from build123d import *
from OCP.BRepFilletAPI import BRepFilletAPI_MakeChamfer

# Parameters (mm, degrees)
SKETCH1_W                  = 50
SKETCH1_H                  = 180
BOSS_EXTRUDE1_DEPTH        = 6
CHAMFER2_SIZE              = 10
F_3_3_3_3_DIAMETER_HOLE1_D = 3.3
BOSS_EXTRUDE3_DEPTH        = 6
CUT_EXTRUDE3_DEPTH         = 2.2
BOSS_EXTRUDE4_DEPTH        = 6
CHAMFER14_SIZE             = 2
CHAMFER16_SIZE             = 7
CHAMFER16_SIZE_2           = 56.79198309
CHAMFER17_SIZE             = 2
SKETCH59_W                 = 21.7
SKETCH59_H                 = 5
BOSS_EXTRUDE5_DEPTH        = 6
CHAMFER19_SIZE             = 5
CUT_EXTRUDE28_DEPTH        = 106.814167745
CHAMFER20_SIZE             = 3
CHAMFER20_SIZE2            = 3.484649721
CUT_EXTRUDE29_DEPTH        = 105.986313168
CHAMFER24_SIZE             = 1
CUT_EXTRUDE31_DEPTH        = 105.986313306
SKETCH66_R                 = 6
BOSS_EXTRUDE6_DEPTH        = 6


with BuildPart() as part:
    # Sketch1 → Boss-Extrude1 (new body)
    with BuildSketch(Plane(origin=(0, 0, 0), x_dir=(1, 0, 0), z_dir=(0, 1, 0))):
        Rectangle(SKETCH1_W, SKETCH1_H)
    extrude(amount=BOSS_EXTRUDE1_DEPTH)

    # Chamfer2
    chamfer2_edges = [part.edges().sort_by_distance(p)[0] for p in [
        (-25, 3, -90),
        (25, 3, -90),
        (25, 3, 90),
        (-25, 3, 90),
    ]]
    chamfer(chamfer2_edges, length=CHAMFER2_SIZE)

    # Ø3.3 (3.3) Diameter Hole1 (through all)
    with Locations(Plane(origin=(0, 6, 0), x_dir=(1, 0, 0), z_dir=(0, 1, 0))):
        with Locations((-19.785088487, 16.105600012), (9.214911513, -56.894399988), (20.785088487, -43.105600012), (-9.214911513, -56.894399988), (-20.785088487, -43.105600012), (19.785088487, 16.105600012), (8.214911513, 29.894399988), (-8.214911513, 29.894399988)):
            Hole(F_3_3_3_3_DIAMETER_HOLE1_D / 2)

    # Sketch52 → Boss-Extrude3 (add, through all)
    with BuildSketch(Plane(origin=(0, 6, 0), x_dir=(1, 0, 0), z_dir=(0, 1, 0))):
        Polygon((40, 33.067924807), (31.85, 24.173760523), (25, 5.3535402), (25, 59.656998575), (28.429823026, 46.856724783), align=None)
        Polygon((-28.429823026, 46.856724783), (-40, 33.067924807), (-31.85, 24.173760523), (-25, 5.3535402), (-25, 59.656998575), align=None)
    extrude(amount=-BOSS_EXTRUDE3_DEPTH)

    # Sketch11 → Cut-Extrude3 (cut)
    with BuildSketch(Plane(origin=(0, 6, 0), x_dir=(1, 0, 0), z_dir=(0, 1, 0))):
        Polygon((23.585088487, -44.722180766), (23.585088487, -41.489019258), (20.785088487, -39.872438504), (17.985088487, -41.489019258), (17.985088487, -44.722180766), (20.785088487, -46.338761519), align=None)
        Polygon((9.214911513, -60.127561496), (12.014911513, -58.510980742), (12.014911513, -55.277819234), (9.214911513, -53.661238481), (6.414911513, -55.277819234), (6.414911513, -58.510980742), align=None)
        Polygon((-6.414911513, -58.510980742), (-9.214911513, -60.127561496), (-12.014911513, -58.510980742), (-12.014911513, -55.277819234), (-9.214911513, -53.661238481), (-6.414911513, -55.277819234), align=None)
        Polygon((-20.785088487, -46.338761519), (-23.585088487, -44.722180766), (-23.585088487, -41.489019258), (-20.785088487, -39.872438504), (-17.985088487, -41.489019258), (-17.985088487, -44.722180766), align=None)
        Polygon((19.785088487, 12.872438504), (22.585088487, 14.489019258), (22.585088487, 17.722180766), (19.785088487, 19.338761519), (16.985088487, 17.722180766), (16.985088487, 14.489019258), align=None)
        Polygon((8.214911513, 26.661238481), (11.014911513, 28.277819234), (11.014911513, 31.510980742), (8.214911513, 33.127561496), (5.414911513, 31.510980742), (5.414911513, 28.277819234), align=None)
        Polygon((-19.785088487, 12.872438504), (-16.985088487, 14.489019258), (-16.985088487, 17.722180766), (-19.785088487, 19.338761519), (-22.585088487, 17.722180766), (-22.585088487, 14.489019258), align=None)
        Polygon((-8.214911513, 26.661238481), (-5.414911513, 28.277819234), (-5.414911513, 31.510980742), (-8.214911513, 33.127561496), (-11.014911513, 31.510980742), (-11.014911513, 28.277819234), align=None)
    extrude(amount=-CUT_EXTRUDE3_DEPTH, mode=Mode.SUBTRACT)

    # Sketch53 → Boss-Extrude4 (add, through all)
    with BuildSketch(Plane(origin=(0, 6, 0), x_dir=(1, 0, 0), z_dir=(0, 1, 0))):
        Polygon((25, -45.989627063), (25, -80), (34, -78.344262241), (46.212964584, -63.789417822), align=None)
        Polygon((-46.212964584, -63.789417822), (-25, -45.989627063), (-25, -80), (-34, -78.344262241), align=None)
    extrude(amount=-BOSS_EXTRUDE4_DEPTH)

    # Chamfer14
    chamfer14_edges = [part.edges().sort_by_distance(p)[0] for p in [
        (-40.106482292, 6, 71.066840031),
        (40.106482292, 6, 71.066840031),
    ]]
    chamfer(chamfer14_edges, length=CHAMFER14_SIZE)

    # Chamfer16
    # the kernel refuses this chamfer: 56.79198309, 7 mm, written as the material it adds along each edge
    with BuildSketch(Plane(origin=(25, 6, 45.989627063), x_dir=(0.6351042832999635, 0, 0.7724264038301901), z_dir=(0, -1, 0))) as chamfer16_piece_1:
        Polygon((CHAMFER16_SIZE * 0.9830242288, -CHAMFER16_SIZE * 0.183475790208), (-CHAMFER16_SIZE_2 * 0.772426403828, -CHAMFER16_SIZE_2 * 0.635104283298), (0, 0), align=None)
    extrude(amount=6)
    with BuildSketch(Plane(origin=(-25, 6, 45.989627063), x_dir=(-0.6351042832999635, 0, 0.7724264038301901), z_dir=(0, -1, 0))) as chamfer16_piece_2:
        Polygon((CHAMFER16_SIZE * 0.9830242288, CHAMFER16_SIZE * 0.183475790208), (-CHAMFER16_SIZE_2 * 0.772426403828, CHAMFER16_SIZE_2 * 0.635104283298), (0, 0), align=None)
    extrude(amount=6)

    # Chamfer17
    chamfer17_edges = [part.edges().sort_by_distance(p)[0] for p in [
        (-34.214911513, 6, -39.962324795),
        (34.214911513, 6, -39.962324795),
    ]]
    chamfer(chamfer17_edges, length=CHAMFER17_SIZE)

    # Sketch59 → Boss-Extrude5 (add, through all)
    with BuildSketch(Plane(origin=(0, 6, 0), x_dir=(1, 0, 0), z_dir=(0, 1, 0))):
        with Locations((0, -92.5)):
            Rectangle(SKETCH59_W, SKETCH59_H)
    extrude(amount=-BOSS_EXTRUDE5_DEPTH)

    # Chamfer19
    chamfer19_edges = [part.edges().sort_by_distance(p)[0] for p in [
        (0, 0, 95),
    ]]
    chamfer(chamfer19_edges, length=CHAMFER19_SIZE)

    # Sketch61 → Cut-Extrude28 (cut, through all)
    with BuildSketch(Plane.XZ):
        Polygon((25, -59.656998575), (15, -90), (25, -80), align=None)
        Polygon((-25, -80), (-25, -59.656998575), (-15, -90), align=None)
    extrude(amount=-CUT_EXTRUDE28_DEPTH, mode=Mode.SUBTRACT)

    # Chamfer20: one chamfer whose edges measure the first distance from different faces: ONE call of the kernel's chamfer builder (chamfer() names one face for all edges)
    chamfer20_edges_1 = [part.edges().sort_by_distance(p)[0] for p in [
        (-40, 2, -33.067924807),
    ]]
    chamfer20_side_1 = [part.faces().sort_by_distance(p)[0] for p in [
        (-35.821197815, 2.933105821, -28.507562458),
    ]]
    chamfer20_edges_2 = [part.edges().sort_by_distance(p)[0] for p in [
        (40, 2, -33.067924807),
    ]]
    chamfer20_side_2 = [part.faces().sort_by_distance(p)[0] for p in [
        (34.214911513, 2, -39.962324795),
    ]]
    chamfer20_edges_3 = [part.edges().sort_by_distance(p)[0] for p in [
        (-46.212964584, 2, 63.789417822),
        (46.212964584, 2, 63.789417822),
    ]]
    chamfer20 = BRepFilletAPI_MakeChamfer(part.part.solid().wrapped)
    for e in chamfer20_edges_1:
        chamfer20.Add(CHAMFER20_SIZE, CHAMFER20_SIZE2, e.wrapped, chamfer20_side_1[0].wrapped)  # the first distance lies on this face
    for e in chamfer20_edges_2:
        chamfer20.Add(CHAMFER20_SIZE, CHAMFER20_SIZE2, e.wrapped, chamfer20_side_2[0].wrapped)  # the first distance lies on this face
    for e in chamfer20_edges_3:
        chamfer20.Add(CHAMFER20_SIZE, e.wrapped)
    add(Compound.cast(chamfer20.Shape()), mode=Mode.REPLACE)

    # Sketch62 → Cut-Extrude29 (cut, through all)
    with BuildSketch(Plane(origin=(0, 6, 0), x_dir=(1, 0, 0), z_dir=(0, 1, 0))):
        with BuildLine():
            Line((15, 90), (25, 59.656998575))
            Line((25, 59.656998575), (28.429823026, 46.856724783))
            add(Edge.make_bspline(
                [(28.429823026, 46.856724783), (20.791344098, 59.90516311), (15, 74.573823319), (15, 90)],
                knots=[0, 0, 0, 0, 1, 1, 1, 1], degree=3))
        make_face()
        with BuildLine():
            Line((-25, 59.656998575), (-28.429823026, 46.856724783))
            add(Edge.make_bspline(
                [(-28.429823026, 46.856724783), (-20.791344098, 59.90516311), (-15, 74.573823319), (-15, 90)],
                knots=[0, 0, 0, 0, 1, 1, 1, 1], degree=3))
            Line((-15, 90), (-25, 59.656998575))
        make_face()
    extrude(amount=-CUT_EXTRUDE29_DEPTH, mode=Mode.SUBTRACT)

    # Chamfer24
    chamfer24_edges = [part.edges().sort_by_distance(p)[0] for p in [
        (0, 0, -90),
    ]]
    chamfer(chamfer24_edges, length=CHAMFER24_SIZE)

    # Sketch64 → Cut-Extrude31 (cut, through all)
    with BuildSketch(Plane(origin=(0, 6, 0), x_dir=(1, 0, 0), z_dir=(0, 1, 0))):
        with BuildLine():
            Line((31.85, 24.173760523), (25, 5.3535402))
            add(Edge.make_bspline(
                [(25, 5.3535402), (25, 9.939182196), (26.103782981, 15.682971222), (29.276150019, 21.364896158), (31.85, 24.173760523)],
                knots=[0, 0, 0, 0, 0.526973907, 1, 1, 1, 1], degree=3))
        make_face()
        with BuildLine():
            Line((-31.85, 24.173760523), (-25, 5.3535402))
            add(Edge.make_bspline(
                [(-25, 5.3535402), (-25, 9.939182196), (-26.103782981, 15.682971222), (-29.276150019, 21.364896158), (-31.85, 24.173760523)],
                knots=[0, 0, 0, 0, 0.526973907, 1, 1, 1, 1], degree=3))
        make_face()
    extrude(amount=-CUT_EXTRUDE31_DEPTH, mode=Mode.SUBTRACT)

    # Sketch66 → Boss-Extrude6 (add)
    with BuildSketch(Plane(origin=(0, 6, 0), x_dir=(1, 0, 0), z_dir=(0, 1, 0))):
        with Locations((29.320888862, -18)):
            Circle(SKETCH66_R)
        with BuildLine():
            ThreePointArc((25, -13.837078017), (26.973287097, -12.478336668), (29.320888862, -12))
            Line((29.320888862, -12), (25, -12))
            Line((25, -12), (25, -13.837078017))
        make_face()
        with BuildLine():
            Line((25, -24), (29.320888862, -24))
            ThreePointArc((29.320888862, -24), (26.973287097, -23.521663332), (25, -22.162921983))
            Line((25, -22.162921983), (25, -24))
        make_face()
        with Locations((-29.320888862, -18)):
            Circle(SKETCH66_R)
        with BuildLine():
            Line((-25, -12), (-29.320888862, -12))
            ThreePointArc((-29.320888862, -12), (-26.973287097, -12.478336668), (-25, -13.837078017))
            Line((-25, -13.837078017), (-25, -12))
        make_face()
        with BuildLine():
            ThreePointArc((-25, -22.162921983), (-26.973287097, -23.521663332), (-29.320888862, -24))
            Line((-29.320888862, -24), (-25, -24))
            Line((-25, -24), (-25, -22.162921983))
        make_face()
    extrude(amount=-BOSS_EXTRUDE6_DEPTH)


solid = part.part
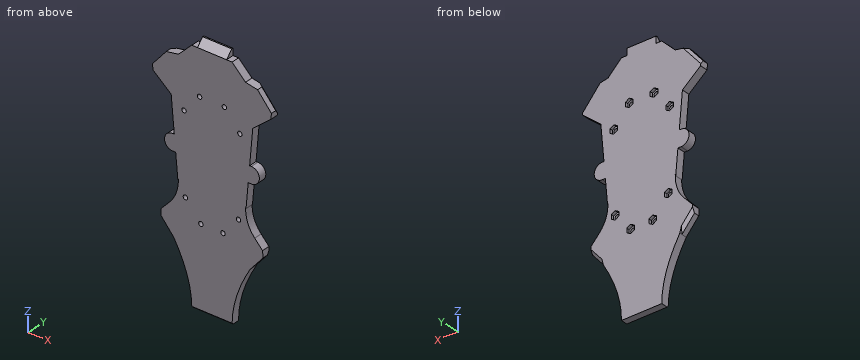
Verification items for the finished model (mm, model axes). Coordinates: 2 decimals unless noted, no trailing zeros. Loops run counter-clockwise (first coordinate to the right, second up) from the corner with the lowest first, then second, coordinate; pieces in that order, holes last. Notation, with made-up numbers: (-5, -36) -> (23, -36) arc R21 cw to (23, -5) -> close; hole circle Ø2 at (80.25, 0.25). An arc over 180 degrees is marked (long way). Write each question's results on one line, items separated by ' | '.
Item 1: Section check B-B, the plane y = 2.5. Count the separate pieces of the cut face and the enclosed holes in it, plus the area to 3 significant figures.
Found:
separate pieces: 1 | enclosed holes: 8 | area: 10,200 mm2
Item 2: Section check C-C, the plane z = 68.5. Enter the section's corners in (x, y).
Found:
outline: (-42.26, 0) -> (42.26, 0) -> (42.26, 4) -> (39.65, 6) -> (-39.65, 6) -> (-42.26, 4) -> close
Item 3: Material ranges on L1, parallel to X at y = 5, z = 60; L2, parallel to Z at x = 33.5, y = 5.5; L3, parallel to Z at x = -22, y = 5, recorded low to high.
Found:
L1: x = -41.7 to -9.44, -8.99 to 8.99, 9.44 to 41.7 | L2: z = -38.48 to -25.97, 13.69 to 22.31, 53.12 to 76.61 | L3: z = -59.38 to -18.06, -14.15 to 40.57, 45.64 to 83
Item 4: Section check A-A, the plane z = 18. Enter the section's corners in (x, y).
Found:
outline: (-35.32, 0) -> (35.32, 0) -> (35.32, 6) -> (-35.32, 6) -> close
Item 5: Gauge pin test, flat ends, axial feed: pin 1 (3 mm diameter, centred on x = -10, z = 57.5, fed in from +Y); pin 2 (2.5 mm diameter, centred on x = -28.5, y = 3.5, fed in from -Z); pin 3 (2 mm diameter, centred on y = 4, z = -43, fed in from +X). Record the tip position at first contact, or that the pin passes through.
Found:
pin 1: stops at y = 3.8 | pin 2: stops at z = -48.91 | pin 3: stops at x = 32.51
